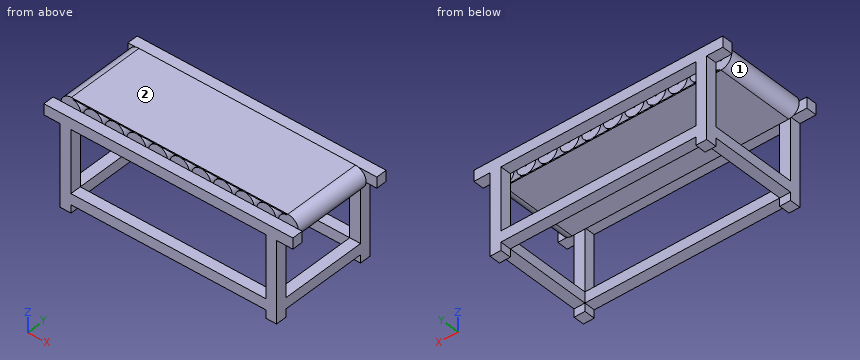
Autodesk Inventor part; units mm, degrees
ref_plane "Work Plane1" through (180, 0, 0) normal (0, -1, 0) x (1, 0, 0)
ref_plane "Work Plane2" through (0, 80, 0) normal (-1, 0, 0) x (0, 0, 1)
ref_plane "Work Plane3" through (-200, 72.5, 34.9541) normal (0, -1, 0) x (1, 0, 0)
sketch "Sketch1" plane through (0, 0, 0) normal (0, 0, 1) x (1, 0, 0)
  line L0 (-200, 100) -> (200, -100) construction
  line L1 (200, 100) -> (-200, -100) construction
  line L2 (-200, 100) -> (-180, 100)
  line L3 (-180, 100) -> (-180, 80)
  line L4 (-180, 80) -> (-200, 80)
  line L5 (-200, 80) -> (-200, 100)
  line L6 (200, 100) -> (180, 100)
  line L7 (180, 100) -> (180, 80)
  line L8 (180, 80) -> (200, 80)
  line L9 (200, 80) -> (200, 100)
  line L10 (200, -100) -> (180, -100)
  line L11 (180, -100) -> (180, -80)
  line L12 (180, -80) -> (200, -80)
  line L13 (200, -80) -> (200, -100)
  line L14 (-200, -100) -> (-180, -100)
  line L15 (-180, -100) -> (-180, -80)
  line L16 (-180, -80) -> (-200, -80)
  line L17 (-200, -80) -> (-200, -100)
  line L18 (-200, 100) -> (-180, 100)
  line L19 (180, 100) -> (200, 100)
  line L20 (-200, -100) -> (-200, -80)
  line L21 (-200, 80) -> (-200, 100)
  line L22 (200, -100) -> (180, -100)
  line L23 (-180, -100) -> (-200, -100)
  line L24 (200, 100) -> (200, 80)
  line L25 (200, -80) -> (200, -100)
  point P0 (0, 0)
  dimension "d0" = 400
  dimension "d1" = 200
  dimension "d2" = 20
  dimension "d3" = 20
  dimension "d4" = 20
  dimension "d5" = 20
  dimension "d6" = 20
  dimension "d7" = 20
  dimension "d8" = 20
  dimension "d9" = 20
extrude "Extrusion1" add sketch "Sketch1" along normal blind 150
sketch "Sketch2" plane through (-200, 80, 0) normal (-1, 0, 0) x (0, 0, 1)
  point P0 (0, -80)
sketch "Sketch3" plane through (-200, 80, 0) normal (-1, 0, 0) x (0, 0, 1)
  line L0 (0, 0) -> (150, 0)
  line L1 (0, -160) -> (150, -160)
  line L2 (34.9541, 0) -> (14.9541, 0)
  line L3 (14.9541, 0) -> (14.9541, -160)
  line L4 (14.9541, -160) -> (34.9541, -160)
  line L5 (34.9541, -160) -> (34.9541, 0)
  point P0 (0, -80)
  dimension "d12" = 20
extrude "Extrusion2" add sketch "Sketch3" against normal blind 20
sketch "Sketch4" plane through (-200, -100, 0) normal (0, -1, 0) x (1, 0, 0)
  line L0 (20, 34.9541) -> (0, 34.9541)
  line L1 (0, 14.9541) -> (20, 14.9541)
  line L2 (380, 0) -> (380, 150)
  line L3 (20, 34.9541) -> (380, 34.9541)
  line L4 (380, 34.9541) -> (380, 14.9541)
  line L5 (380, 14.9541) -> (20, 14.9541)
  line L6 (20, 14.9541) -> (20, 34.9541)
  point P0 (200, 0)
extrude "Extrusion3" add sketch "Sketch4" against normal blind 20
ref_plane "Work Plane1" through (180, 0, 0) normal (0, -1, 0) x (1, 0, 0)
mirror "Mirror1" about plane through (180, 0, 0) normal (0, -1, 0) of "Extrusion3"
ref_plane "Work Plane2" through (0, 80, 0) normal (-1, 0, 0) x (0, 0, 1)
mirror "Mirror2" about plane through (0, 80, 0) normal (-1, 0, 0) of "Extrusion2"
sketch "Sketch5" plane through (180, -100, 0) normal (0, -1, 0) x (1, 0, 0)
  line L0 (-380, 14.9541) -> (-360, 14.9541)
  line L1 (-360, 34.9541) -> (-380, 34.9541)
  line L2 (-360, 0) -> (-360, 14.9541)
  line L3 (-380, 0) -> (-360, 0)
  line L4 (-380, 150) -> (-360, 150)
  line L5 (-410, 150) -> (50, 150)
  line L6 (50, 150) -> (50, 170)
  line L7 (50, 170) -> (-410, 170)
  line L8 (-410, 170) -> (-410, 150)
  line L9 (-380, 0) -> (-380, 150)
  line L10 (20, 0) -> (20, 150)
  point P0 (-180, 0)
  dimension "d17" = 14.9541
  dimension "d20" = 460
  dimension "d21" = 20
  dimension "d22" = 30
extrude "Extrusion4" add sketch "Sketch5" against normal blind 20 contours L5 L8 L7 L6 L4
mirror "Mirror3" about plane through (180, 0, 0) normal (0, -1, 0) of "Extrusion4"
sketch "Sketch6" plane through (-200, 80, 34.9541) normal (0, -1, 0) x (1, 0, 0)
  point P0 (200, -34.9541)
ref_plane "Work Plane3" through (-200, 72.5, 34.9541) normal (0, -1, 0) x (1, 0, 0)
sketch "Sketch7" plane through (-200, 72.5, 34.9541) normal (0, -1, 0) x (1, 0, 0)
  circle A0 centre (-2.9279, 124.2812) radius 17.5
  circle A1 centre (-2.9279, 124.2812) radius 17.5
  point P0 (200, -34.9541)
  dimension "d27" = 35
extrude "Extrusion5" add sketch "Sketch7" along normal blind 145
pattern_linear "Rectangular Pattern1" count 11 spacing 40 along (1, 0, 0) of "Extrusion5"
sketch "Sketch11" plane through (-200, 80, 34.9541) normal (0, -1, 0) x (1, 0, 0)
  circle A0 centre (-2.9279, 124.2812) radius 17.5
  circle A1 centre (-2.9279, 124.2812) radius 2.5
  point P0 (200, -34.9541)
  dimension "d33" = 5
extrude "Extrusion6" add sketch "Sketch11" along normal up to surface (160 mm away) contours A1
pattern_linear "Rectangular Pattern2" count 11 spacing 40 along (1, 0, 0) of "Extrusion6"
ref_plane "Work Plane5" through (-200, -72.5, 34.9541) normal (0, 1, 0) x (1, 0, 0)
sketch "Sketch20" plane through (-200, -72.5, 34.9541) normal (0, 1, 0) x (1, 0, 0)
  circle A0 centre (-2.9279, -124.2812) radius 2.5
  arc A1 (-2.9279, -106.7812) -> (-2.9279, -141.7812) centre (-2.9279, -124.2812) ccw
  circle A2 centre (397.0721, -124.2812) radius 2.5
  line L0 (-2.9279, -141.7812) -> (397.0721, -141.7812)
  line L1 (-2.9279, -106.7812) -> (397.0721, -106.7812)
  circle A3 centre (397.0721, -124.2812) radius 17.5
  arc A4 (397.0721, -141.7812) -> (397.0721, -106.7812) centre (397.0721, -124.2812) ccw
  circle A5 centre (397.0721, -124.2812) radius 17.5
  line L2 (397.0721, -143.7812) -> (-2.9279, -143.7812)
  arc A6 (-2.9279, -104.7812) -> (-2.9279, -143.7812) centre (-2.9279, -124.2812) ccw
  line L3 (-2.9279, -104.7812) -> (397.0721, -104.7812)
  arc A7 (397.0721, -143.7812) -> (397.0721, -104.7812) centre (397.0721, -124.2812) ccw
  point P0 (200, 34.9541)
  dimension "d68" = 35
  dimension "d69" = 2
extrude "Extrusion7" add sketch "Sketch20" along normal blind 145 contours L2 A6 L3 A7
properties part number "Traka"
Source: CAD feature listing. Evaluate the final solid. Frame: model axes, mm. Face numbers are marked on the shaded views. Round coordinates to 2 decimals unless told otherwise and drop trailing zeros. Write each loop counter-clockwise with the first axis right and the second up, starting at its lowest first coordinate (ties: lowest second). Pieces come first, ordered by that corner, then holes. Notation, with made-up numbers: M 72.5,30 L 104.5,30 A37 cw 104.5,69 Z; hole C 21.5,26 d11. An arc over 180 degrees is marked long. One line per item, written item: value. Start each with the question number.
Item 1: Pin query (flat end, axial travel): pin 1 (10 mm diameter, centred on y = -18, z = 28.5, fed in from -X); pin 2 (10 mm diameter, centred on x = 168, z = 141, fed in from +Y); pin 3 (22 mm diameter, centred on x = 187, y = -28, fed in from -Z). Return the tip coordinate at first contact, or that it passes through.
Item 2: Ray query, L1, parallel to Z at x = -31.5, y = -20; L2, parallel to Z at x = 32, y = 84; L3, parallel to Z at x = 18, y = -48.5. Return the intervals inside material, ascending. Write a range as from..to.
Item 3: Section query A-A (z = 92). Return the cut outline in (x, y).
Item 4: Section query D-D (x = 49.5). Return the cut outline in (y, z), plus the area to 3 significant figures.
Item 5: Mould query, pull axis Y, two halves, no side actions, for the marked faces 1 and 2. Classes: pulls with the +Y half, pulls with the -Y half, needs draft (parallel to the pull), parting line crosses it, or undercut.
Item 6: Section query B-B (x = 108). Return the cut outline in (y, z).
Result set:
1. pin 1: stops at x = -200
1. pin 2: stops at y = 72.5
1. pin 3: stops at z = 14.95
2. L1: z = 139.74..141.74, 145.98..172.49, 176.74..178.74
2. L2: z = 14.95..34.95, 150..170
2. L3: z = 139.74..141.74, 176.74..178.74
3. outline: M -200,-100 L -180,-100 L -180,-80 L -200,-80 Z; M -200,80 L -180,80 L -180,100 L -200,100 Z; M 180,-100 L 200,-100 L 200,-80 L 180,-80 Z; M 180,80 L 200,80 L 200,100 L 180,100 Z
4. outline: M -100,14.95 L -80,14.95 L -80,34.95 L -100,34.95 Z; M -100,150 L -80,150 L -80,170 L -100,170 Z; M -72.5,139.74 L 72.5,139.74 L 72.5,141.74 L -72.5,141.74 Z; M -72.5,146.91 L 72.5,146.91 L 72.5,171.56 L -72.5,171.56 Z; M -72.5,176.74 L 72.5,176.74 L 72.5,178.74 L -72.5,178.74 Z; M 80,14.95 L 100,14.95 L 100,34.95 L 80,34.95 Z; M 80,150 L 100,150 L 100,170 L 80,170 Z
4. area: 5,750 mm²
5. face 1: undercut
5. face 2: needs draft
6. outline: M -100,14.95 L -80,14.95 L -80,34.95 L -100,34.95 Z; M -100,150 L -80,150 L -80,170 L -100,170 Z; M -72.5,139.74 L 72.5,139.74 L 72.5,141.74 L -72.5,141.74 Z; M -72.5,144.27 L 72.5,144.27 L 72.5,174.2 L -72.5,174.2 Z; M -72.5,176.74 L 72.5,176.74 L 72.5,178.74 L -72.5,178.74 Z; M 80,14.95 L 100,14.95 L 100,34.95 L 80,34.95 Z; M 80,150 L 100,150 L 100,170 L 80,170 Z
